Read the model definition and answer for the solid it produces. Units are mm, in the model's axes. A direction names the side the tool comes from. Coordinates: 2 decimals unless noted, no trailing zeros. Order: outer loops, then holes, each group sorted by start corner. A loop starts at its lowest first (then second) coordinate and runs counter-clockwise, first axis right, second up. Notation, with made-up numbers: M 66,17 L 114,17 A16 ccw 114,48 Z; hole C 43,46.5 d6. An arc over 180 degrees is marked long. Write each question's results on one line, items separated by ' | '.
```python
from build123d import *

# Parameters (mm, degrees)
F1_DEPTH = 100
F2_SIZE2 = 115.4700538379
F2_SIZE  = 200
F3_R     = 50
F4_R     = 10
F5_DEPTH = 100


with BuildPart() as f1:
    # F0 (on Front) → F1 (new body, symmetric)
    with BuildSketch(Plane.XZ):
        with BuildLine():
            Line((-72, 277.65), (-72, 0))
            Line((-72, 0), (-68, 0))
            Line((-68, 0), (-68, 280))
            Line((-68, 280), (72, 280))
            Line((72, 280), (72, 0))
            Line((72, 0), (76, 0))
            Line((76, 0), (76, 277.65))
            ThreePointArc((76, 277.65), (74.1401280605, 282.1401280605), (69.65, 284))
            Line((69.65, 284), (-65.65, 284))
            ThreePointArc((-65.65, 284), (-70.1401280605, 282.1401280605), (-72, 277.65))
        make_face()
    extrude(amount=F1_DEPTH, both=True)

    # F2
    f2_edges = [f1.edges().sort_by_distance(p)[0] for p in [
        (74, -100, 0),
        (-70, -100, 0),
    ]]
    f2_side = f1.faces().sort_by_distance((-68.797501, -100, 138.825))[0]
    chamfer(f2_edges, length=F2_SIZE, length2=F2_SIZE2, reference=f2_side)

    # F3
    f3_edges = [f1.edges().sort_by_distance(p)[0] for p in [
        (74, -100, 200),
        (-70, -100, 200),
        (74, 15.470054, 0),
        (-70, 15.470054, 0),
        (-70, 100, 0),
        (74, 100, 0),
    ]]
    fillet(f3_edges, radius=F3_R)

    # F4 (on Right) → F5 (cut, symmetric)
    with BuildSketch(Plane.YZ):
        with Locations((50, 40)):
            Circle(F4_R)
    extrude(amount=F5_DEPTH, both=True, mode=Mode.SUBTRACT)


solid = f1.part
```
(1) For faces 1 (the flat face through (74, -45.5, 105.6)), 2 (the flat face through (1, -1, 280)), determine the directions among +Z, -Z, +X, -X, +Y, -Y from which every point of the face is accessible in a straight line to the end or side of a thin tool.
Conclusion:
face 1: -Z, +X, -X, -Y | face 2: -Z, +Y, -Y
(2) Given pin 1 (4 mm diameter, centred on x = 55, y = 0, fed in from -Z); pin 2 (23 mm diameter, centred on y = 50, z = 40, fed in from +X), each flat-ended and moving along its own axis, determine where each tip first touches the part or whether it passes through.
Conclusion:
pin 1: z = 280 | pin 2: x = 76
(3) The part is cut by section D-D, the plane x = -1. Write down the section's boundary in (y, z), then the cut area to 3 significant figures.
Conclusion:
outline: M -100,280 L 100,280 L 100,284 L -100,284 Z | area: 800 mm²
(4) The mould has two halves that part along X. Classify faces 3 (the flat face through (-72, 21, 172)), 4 (the flat face through (-68, 21, 169)), 5 (the flat face through (76, 21, 168)): pulls with the +X half, pulls with the -X half, needs draft (parallel to the pull), parting line crosses it, or undercut.
Conclusion:
face 3: pulls with the -X half | face 4: undercut | face 5: pulls with the +X half
(5) Straight lines are drawn through the part: line 1 (X direction, y = -25, z = 192.5); line 2 (Z direction, x = 1, y = 26). For each, find the intervals that lie inside material, in ascending order.
Conclusion:
line 1: -72 to -68, 72 to 76 | line 2: 280 to 284
(6) The part is cut by section C-C, the plane z = 144. Write down the section's boundary in (x, y).
Conclusion:
outline: M -72,-67.67 L -68,-67.67 L -68,100 L -72,100 Z; M 72,-67.67 L 76,-67.67 L 76,100 L 72,100 Z
(7) The part is cut by section B-B, the plane y = 21. Write down the section's boundary in (x, z), then the cut area to 3 significant figures.
Conclusion:
outline: M -72,5.78 L -68,5.78 L -68,280 L 72,280 L 72,5.78 L 76,5.78 L 76,277.65 A6.35 ccw 69.65,284 L -65.65,284 A6.35 ccw -72,277.65 Z | area: 2,770 mm²
(8) The part is cut by section A-A, the plane z = 21.5. Write down the section's boundary in (x, y).
Conclusion:
outline: M -72,3.26 L -68,3.26 L -68,91.08 L -72,91.08 Z; M 72,3.26 L 76,3.26 L 76,91.08 L 72,91.08 Z
